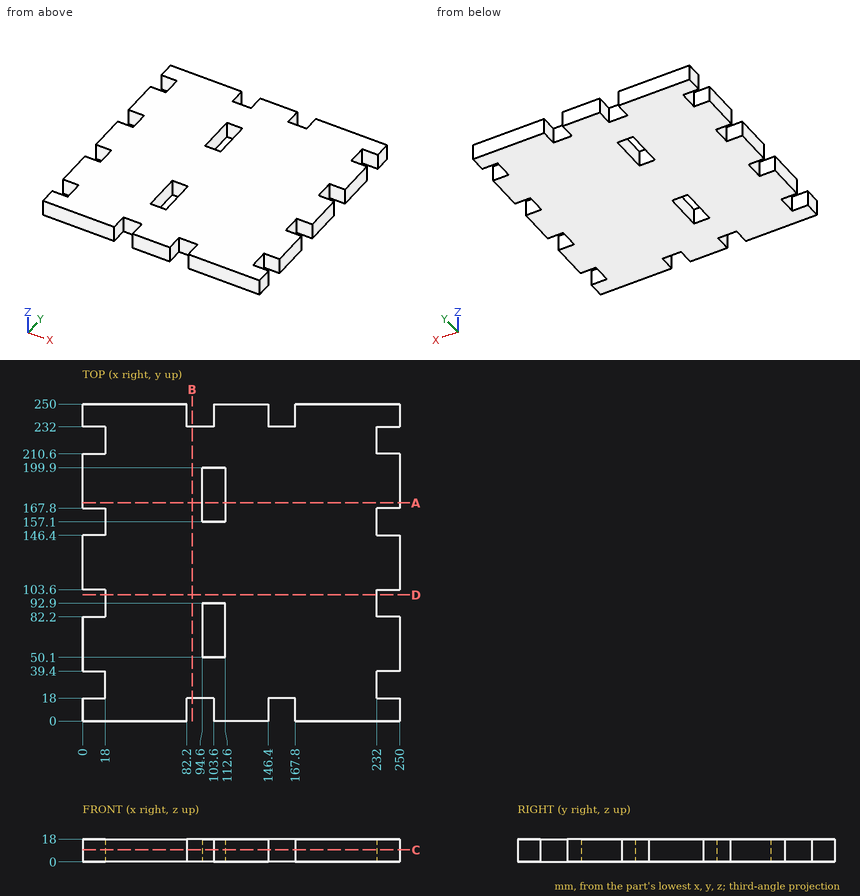
Could you check a few things on this drawing? It's one solid part, dimensions in mm from its lowest x, y, z. Coordinates: 2 decimals unless noted, no trailing zeros. Order: outer loops, then holes, each group sorted by start corner. A loop starts at its lowest first (then second) coordinate and runs counter-clockwise, first axis right, second up. Notation, with made-up numbers: (59, -20.5) - (117, -20.5) arc R29 ccw to (117, 11.5) - close; hole circle Ø2 at (35, 24.25). An arc over 180 degrees is marked (long way). One line per question, with ' | ' between items. Start each with the question number.
1. If we section it at C-C (z = 9.5): Give the number of separate pieces and of enclosed holes in the cut face, and give its area (3 significant figures).
2. Please list where these lines run through material, in increasing order: line 1 along Y through (x, z) = (11, 13.5); line 2 along Y through (x, z) = (104.5, 13.5); line 3 along X through (y, z) = (197, 12.5). Write a range as [from, to].
3. If we section it at B-B (x = 86.5): Write out the boundary of the cut face in (y, z).
4. I'm going to push flat-ended pins straight in: pin 1 Ø9 at (x, z) = (11.5, 9.5) entering from -Y; pin 2 Ø1.5 at (x, z) = (88.5, 4.5) entering from -Y; pin 3 Ø1 at (y, z) = (84.5, 11.5) entering from -X; pin 4 Ø5.5 at (y, z) = (152.5, 4.5) entering from +X. Where does each tip first touch, or does it pass through?
5. If we section it at A-A (y = 172): Write out the boundary of the cut face in (x, z), and give its area (3 significant figures).
Model answer:
1) separate pieces: 1 | enclosed holes: 2 | area: 56,300 mm²
2) line 1: y = [0, 18], [39.4, 82.2], [103.6, 146.4], [167.8, 210.6], [232, 250] | line 2: y = [0, 50.1], [92.9, 157.1], [199.9, 250] | line 3: x = [0, 94.6], [112.6, 250]
3) outline: (18, 0) - (232, 0) - (232, 18) - (18, 18) - close
4) pin 1: stops at y = 0 | pin 2: stops at y = 18 | pin 3: stops at x = 18 | pin 4: stops at x = 232
5) outline: (0, 0) - (94.6, 0) - (94.6, 18) - (0, 18) - close; (112.6, 0) - (250, 0) - (250, 18) - (112.6, 18) - close | area: 4,180 mm²
